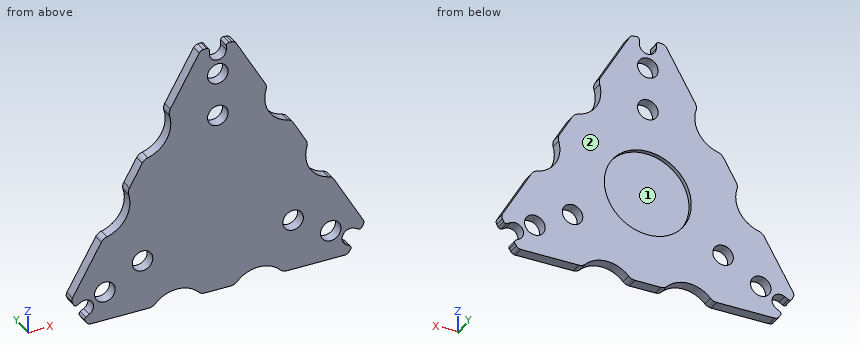
from build123d import *

# Parameters (mm, degrees)
F0_R     = 5.9944
F0_R_2   = 25.4
F1_DEPTH = 6.35
F2_DEPTH = 2.54
F3_R     = 1.524
F4_R     = 3.048
F5_R     = 5.08


with BuildPart() as f1:
    # F0 (on Front) → F1 (new body)
    with BuildSketch(Plane.XZ):
        with BuildLine():
            ThreePointArc((4.951105, 89.398002), (0, 84.582), (-4.951105, 89.398002))
            Line((-4.951105, 89.398002), (-4.951105, 93.506112))
            Line((-4.951105, 93.506112), (-10.074773, 93.093531))
            Line((-10.074773, 93.093531), (-28.89515, 60.495681))
            ThreePointArc((-28.89515, 60.495681), (-29.775746, 44.776954), (-42.948265, 36.154973))
            Line((-42.948265, 36.154973), (-52.785257, 19.116802))
            ThreePointArc((-52.785257, 19.116802), (-53.665853, 3.398075), (-66.838372, -5.223907))
            Line((-66.838372, -5.223907), (-85.658749, -37.821756))
            Line((-85.658749, -37.821756), (-83.505709, -42.363937))
            Line((-83.505709, -42.363937), (-79.896493, -40.411218))
            ThreePointArc((-79.896493, -40.411218), (-73.250161, -42.291), (-74.945388, -48.986784))
            Line((-74.945388, -48.986784), (-78.4411, -51.136097))
            Line((-78.4411, -51.136097), (-75.652926, -55.177362))
            Line((-75.652926, -55.177362), (-37.87309, -55.177362))
            ThreePointArc((-37.87309, -55.177362), (-23.890107, -48.17503), (-9.907124, -55.177362))
            Line((-9.907124, -55.177362), (9.907124, -55.177362))
            ThreePointArc((9.907124, -55.177362), (23.890107, -48.17503), (37.87309, -55.177362))
            Line((37.87309, -55.177362), (75.806581, -55.177362))
            Line((75.806581, -55.177362), (78.4411, -51.136097))
            Line((78.4411, -51.136097), (74.945388, -48.986784))
            ThreePointArc((74.945388, -48.986784), (73.250161, -42.291), (79.896493, -40.411218))
            Line((79.896493, -40.411218), (83.505709, -42.363937))
            Line((83.505709, -42.363937), (85.688288, -38.061744))
            Line((85.688288, -38.061744), (66.721542, -5.210377))
            ThreePointArc((66.721542, -5.210377), (53.665853, 3.398075), (52.73856, 19.00886))
            Line((52.73856, 19.00886), (42.831435, 36.168502))
            ThreePointArc((42.831435, 36.168502), (29.775746, 44.776954), (28.848452, 60.387739))
            Line((28.848452, 60.387739), (9.958534, 93.106037))
            Line((9.958534, 93.106037), (4.951105, 93.506112))
            Line((4.951105, 93.506112), (4.951105, 89.398002))
        make_face()
        with Locations((-65.95814, -38.08095)):
            Circle(F0_R, mode=Mode.SUBTRACT)
        with Locations((-43.961095, -25.38095)):
            Circle(F0_R, mode=Mode.SUBTRACT)
        Circle(F0_R_2, mode=Mode.SUBTRACT)
        with Locations((65.95814, -38.08095)):
            Circle(F0_R, mode=Mode.SUBTRACT)
        with Locations((43.961095, -25.38095)):
            Circle(F0_R, mode=Mode.SUBTRACT)
        with Locations((0, 50.7619)):
            Circle(F0_R, mode=Mode.SUBTRACT)
        with Locations((0, 76.1619)):
            Circle(F0_R, mode=Mode.SUBTRACT)
        Circle(F0_R_2)
    extrude(amount=F1_DEPTH)

    # F0 (on Front) → F2 (cut)
    with BuildSketch(Plane.XZ):
        Circle(F0_R_2)
    extrude(amount=F2_DEPTH, mode=Mode.SUBTRACT)

    # F3
    f3_edges = [f1.edges().sort_by_distance(p)[0] for p in [
        (83.505709, -3.175, -42.363937),
        (78.4411, -3.175, -51.136097),
        (4.951105, -3.175, 93.506112),
        (-4.951105, -3.175, 93.506112),
        (-83.505709, -3.175, -42.363937),
        (-78.4411, -3.175, -51.136097),
    ]]
    fillet(f3_edges, radius=F3_R)

    # F4
    f4_edges = [f1.edges().sort_by_distance(p)[0] for p in [
        (-85.658749, -3.175, -37.821756),
        (-75.652926, -3.175, -55.177362),
        (75.806581, -3.175, -55.177362),
        (85.688288, -3.175, -38.061744),
        (9.958534, -3.175, 93.106037),
        (-10.074773, -3.175, 93.093531),
    ]]
    fillet(f4_edges, radius=F4_R)

    # F5
    f5_edges = [f1.edges().sort_by_distance(p)[0] for p in [
        (28.848452, -3.175, 60.387739),
        (42.831435, -3.175, 36.168502),
        (52.73856, -3.175, 19.00886),
        (66.721542, -3.175, -5.210377),
        (37.87309, -3.175, -55.177362),
        (9.907124, -3.175, -55.177362),
        (-9.907124, -3.175, -55.177362),
        (-37.87309, -3.175, -55.177362),
        (-66.838372, -3.175, -5.223907),
        (-52.785257, -3.175, 19.116802),
        (-42.948265, -3.175, 36.154973),
        (-28.89515, -3.175, 60.495681),
    ]]
    fillet(f5_edges, radius=F5_R)


solid = f1.part
Here's how the part is built. I have some questions about the finished solid (model axes, mm). Face numbers are marked on the shaded views. Coordinates: 2 decimals unless noted, no trailing zeros. Write each loop counter-clockwise with the first axis right and the second up, starting at its lowest first coordinate (ties: lowest second). Pieces come first, ordered by that corner, then holes.
1) Thinking about a two-plate mould opening in X: for the marked faces 1 and 2, which applies, +X half, -X half, draft (parallel to the pull), parting line (faces both ways), or undercut?
Filled in:
face 1: undercut
face 2: draft
2) If we section it at A-A (x = 0): List the corners of the cut face in (y, z) for me, plus the area to 3 significant figures.
Filled in:
outline: (-6.35, -55.18) - (0, -55.18) - (0, -25.4) - (-2.54, -25.4) - (-2.54, 25.4) - (0, 25.4) - (0, 44.77) - (-6.35, 44.77) - close; (-6.35, 56.76) - (0, 56.76) - (0, 70.17) - (-6.35, 70.17) - close; (-6.35, 82.16) - (0, 82.16) - (0, 84.58) - (-6.35, 84.58) - close
area: 606 mm2
3) I'm going to push flat-ended pins straight in: pin 1 (11 mm diameter, centred on x = -43.96, z = -25.38, fed in from -Y); pin 2 (0.7 mm diameter, centred on y = -3, z = 91, fed in from -X); pin 3 (1 mm diameter, centred on x = 42, y = -3.5, fed in from +Z); pin 4 (2.5 mm diameter, centred on y = -2.5, z = 90.5, fed in from +X). Where does each tip first touch, or does it pass through?
Filled in:
pin 1: passes through
pin 2: stops at x = -11.49
pin 3: stops at z = 36.31
pin 4: stops at x = 12.18
4) If we section it at B-B (z = -23.5): List the corners of the cut face in (x, y) for me.
Filled in:
outline: (-77.39, -6.35) - (-49.65, -6.35) - (-49.65, 0) - (-77.39, 0) - close; (-38.27, -6.35) - (38.27, -6.35) - (38.27, 0) - (9.64, 0) - (9.64, -2.54) - (-9.64, -2.54) - (-9.64, 0) - (-38.27, 0) - close; (49.65, -6.35) - (77.28, -6.35) - (77.28, 0) - (49.65, 0) - close
5) If I drill on line 1 (Z direction, x = 0, y = -1.2); line 2 (X direction, y = -1, z = 59.5); line 3 (X direction, y = -2.25, z = -26), over which ranges is the centre line in solid material (lowest first)?
Filled in:
line 1: z = -55.18 to -25.4, 25.4 to 44.77, 56.76 to 70.17, 82.16 to 84.58
line 2: x = -28.37 to 28.34
line 3: x = -78.83 to -49.92, -38 to 38, 49.92 to 78.72
6) If we section it at C-C (x = 62): List the corners of the cut face in (y, z) for me.
Filled in:
outline: (-6.35, -55.18) - (0, -55.18) - (0, -42.58) - (-6.35, -42.58) - close; (-6.35, -33.58) - (0, -33.58) - (0, -3.96) - (-6.35, -3.96) - close
7) If we section it at D-D (z = 48.5): List the corners of the cut face in (x, y) for me.
Filled in:
outline: (-28.17, -6.35) - (-5.55, -6.35) - (-5.55, 0) - (-28.17, 0) - close; (5.55, -6.35) - (28.17, -6.35) - (28.17, 0) - (5.55, 0) - close
